Read the model definition and answer for the solid it produces. Units are mm, in the model's axes. A direction names the side the tool comes from. Give positions to 0.01 mm unless a question says otherwise; leave off trailing zeros. Loops run counter-clockwise (first coordinate to the right, second up) from the corner with the lowest first, then second, coordinate; pieces in that order, holes last. Notation, with made-up numbers: (20.5, -2) - (44.5, -2) arc R12 ccw to (44.5, 15) - close; hole circle Ø7 at (-37.75, 21.25). An arc over 180 degrees is marked (long way). Write item = value, one per line.
```python
from build123d import *

# Parameters (mm, degrees)
BOSS_EXTRUDE1_DEPTH = 1.5875


with BuildPart() as part:
    # Sketch40 → Boss-Extrude1 (new body)
    with BuildSketch(Plane(origin=(-456.955039877, 178.120588246, -67.48659487), x_dir=(-0.1270105543825624, 0.04950857893190621, 0.9906650390962515), z_dir=(-0.9230204054682253, 0.35979237176022855, -0.13631867191409483))):
        Polygon((-143.227084656, 906.623268698), (-170.661347691, 874.056453533), (-74.641427067, 839.002915601), (-74.641427067, 881.585027318), align=None)
        with BuildLine():
            Line((-115.271977523, 886.304578524), (-109.11217167, 884.055847358))
            ThreePointArc((-109.11217167, 884.055847358), (-105.459844174, 871.54470512), (-116.313665717, 864.329254051))
            Line((-116.313665717, 864.329254051), (-122.47347157, 866.577985217))
            ThreePointArc((-122.47347157, 866.577985217), (-126.125799067, 879.089127455), (-115.271977523, 886.304578524))
        make_face(mode=Mode.SUBTRACT)
    extrude(amount=BOSS_EXTRUDE1_DEPTH)


with BuildPart() as body_2:
    # Mirror2: mirrored copy
    add(part.part.mirror(Plane(origin=(0, 0, 0), x_dir=(0, 0, 1), z_dir=(1, 0, 0))))


solid = body_2.part
```
1) Find the intervals of material crossed by probe 1 along X at (y, z) = (980, -171); probe 2 along X at (y, z) = (997, -192), in increasing order.
Output:
probe_1 = 129.1 to 130.82
probe_2 = 119.37 to 121.09
2) Each of these flat-tipped pins is pushed along its axis until it touches: P1, Ø10, axis at y = 995, z = -156, coming from the +X side; P2, Ø12, axis at x = 114.5, y = 1001.5, coming from the -Z side; P3, Ø4, axis at y = 991, z = -161, coming from the +X side. Where does it stop, or does it pass through?
Output:
P1 = 129.27
P2 = -227.19
P3 = 128.84
3) A tool of negligible diameter and unlimited length cuts with its end or side. For faces 1 (the face through (127.694, 985.39, -172.004)), 2 (the face through (128.21, 978.84, -185.83)), 3 (the face through (114.33, 1000.4, -222.88)), from which of +Z, -Z, +X, -X, +Y, -Y can it reach the whole face along a straight path? Write none if from no direction.
Output:
face_1 = none
face_2 = -X, +Y
face_3 = -Z, -X, +Y
4) The mould has two halves that part along Z. Classify faces 4 (the face through (128.323, 979.242, -189.875)), 5 (the face through (126.86, 978.67, -189.66)), 6 (the face through (122.447, 991.046, -192.606)), 7 (the face through (121.935, 997.599, -178.781)): pulls with the +Z half, pulls with the -Z half, needs draft (parallel to the pull), parting line crosses it, or undercut.
Output:
face_4 = pulls with the -Z half
face_5 = pulls with the +Z half
face_6 = undercut
face_7 = undercut
5) A cutting plane is placed at B-B on z = -160.5. Determine the outline of the cut face in (x, y).
Output:
outline = (122.3, 1001.41) - (137.77, 961.73) - (139.29, 962.24) - (123.82, 1001.92) - close
6) A cutting plane is placed at A-A on y = 1013. Determine the outline of the cut face in (x, z).
Output:
outline = (110.22, -211.73) - (111.83, -212.44) - (113.92, -198.28) - (111.95, -200.01) - close
